Can you work these out from the model? Positions are in its coordinate system, mm. Give positions to 0.01 mm unless a question says otherwise; leave off trailing zeros. Write each loop counter-clockwise with the first axis right and the second up, starting at its lowest first coordinate (ties: lowest second). Pieces come first, ordered by that corner, then holes.
```python
from build123d import *
from OCP.BRepFilletAPI import BRepFilletAPI_MakeChamfer

# Parameters (mm, degrees)
SKETCH1_W           = 990
SKETCH1_H           = 1658
BOSS_EXTRUDE1_DEPTH = 42
SKETCH2_W           = 958
SKETCH2_H           = 1626
CUT_EXTRUDE1_DEPTH  = 2
SKETCH3_W           = 968
SKETCH3_H           = 1636
CUT_EXTRUDE2_DEPTH  = 1932.492687017
SKETCH4_W           = 968
SKETCH4_H           = 1636
SKETCH4_W_2         = 946
SKETCH4_H_2         = 1614
BOSS_EXTRUDE2_DEPTH = 1
CUT_EXTRUDE3_START  = -4
SKETCH5_W           = 980
SKETCH5_H           = 1648
CUT_EXTRUDE3_DEPTH  = 3
CHAMFER1_SIZE       = 3
CHAMFER1_SIZE2      = 5.196152423


with BuildPart() as part:
    # Sketch1 → Boss-Extrude1 (new body)
    with BuildSketch(Plane.XY):
        with Locations((495, 829)):
            Rectangle(SKETCH1_W, SKETCH1_H)
    extrude(amount=BOSS_EXTRUDE1_DEPTH)

    # Sketch2 → Cut-Extrude1 (cut)
    with BuildSketch(Plane.XY.offset(42)):
        with Locations((495, 829)):
            Rectangle(SKETCH2_W, SKETCH2_H)
    extrude(amount=-CUT_EXTRUDE1_DEPTH, mode=Mode.SUBTRACT)

    # Sketch3 → Cut-Extrude2 (cut, through all)
    with BuildSketch(Plane.XY.offset(40)):
        with Locations((495, 829)):
            Rectangle(SKETCH3_W, SKETCH3_H)
    extrude(amount=-CUT_EXTRUDE2_DEPTH, mode=Mode.SUBTRACT)

    # Sketch4 → Boss-Extrude2 (add)
    with BuildSketch(Plane.XY.offset(7)):
        with Locations((495, 829)):
            Rectangle(SKETCH4_W, SKETCH4_H)
        with Locations((495, 829)):
            Rectangle(SKETCH4_W_2, SKETCH4_H_2, mode=Mode.SUBTRACT)
    extrude(amount=BOSS_EXTRUDE2_DEPTH)

    # Sketch5 → Cut-Extrude3 (cut)
    with BuildSketch(Plane(origin=(0, 0, 0), x_dir=(-1, 0, 0), z_dir=(0, 0, -1)).offset(CUT_EXTRUDE3_START)):
        with Locations((-495, 829)):
            Rectangle(SKETCH5_W, SKETCH5_H)
    extrude(amount=-CUT_EXTRUDE3_DEPTH, mode=Mode.SUBTRACT)

    # Chamfer1: one chamfer whose edges measure the first distance from different faces: ONE call of the kernel's chamfer builder (chamfer() names one face for all edges)
    chamfer1_edges_1 = [part.edges().sort_by_distance(p)[0] for p in [
        (495, 1647, 0),
    ]]
    chamfer1_side_1 = [part.faces().sort_by_distance(p)[0] for p in [
        (495, 1647, 2),
    ]]
    chamfer1_edges_2 = [part.edges().sort_by_distance(p)[0] for p in [
        (979, 829, 0),
    ]]
    chamfer1_side_2 = [part.faces().sort_by_distance(p)[0] for p in [
        (979, 829, 2),
    ]]
    chamfer1_edges_3 = [part.edges().sort_by_distance(p)[0] for p in [
        (495, 11, 0),
    ]]
    chamfer1_side_3 = [part.faces().sort_by_distance(p)[0] for p in [
        (495, 11, 2),
    ]]
    chamfer1_edges_4 = [part.edges().sort_by_distance(p)[0] for p in [
        (11, 829, 0),
    ]]
    chamfer1_side_4 = [part.faces().sort_by_distance(p)[0] for p in [
        (11, 829, 2),
    ]]
    chamfer1 = BRepFilletAPI_MakeChamfer(part.part.solid().wrapped)
    for e in chamfer1_edges_1:
        chamfer1.Add(CHAMFER1_SIZE, CHAMFER1_SIZE2, e.wrapped, chamfer1_side_1[0].wrapped)  # the first distance lies on this face
    for e in chamfer1_edges_2:
        chamfer1.Add(CHAMFER1_SIZE, CHAMFER1_SIZE2, e.wrapped, chamfer1_side_2[0].wrapped)  # the first distance lies on this face
    for e in chamfer1_edges_3:
        chamfer1.Add(CHAMFER1_SIZE, CHAMFER1_SIZE2, e.wrapped, chamfer1_side_3[0].wrapped)  # the first distance lies on this face
    for e in chamfer1_edges_4:
        chamfer1.Add(CHAMFER1_SIZE, CHAMFER1_SIZE2, e.wrapped, chamfer1_side_4[0].wrapped)  # the first distance lies on this face
    add(Compound.cast(chamfer1.Shape()), mode=Mode.REPLACE)


solid = part.part
```
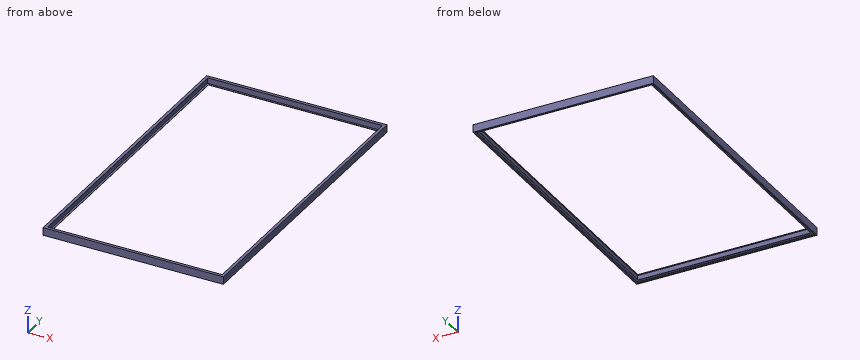
1) Suppose I cut it at B-B on y = 1087. Write out the boundary of the cut face in (x, z), plus the area to 3 significant figures.
Values follow:
outline: (0, 0) - (5.8, 0) - (11, 3) - (11, 4) - (5, 4) - (5, 7) - (22, 7) - (22, 8) - (11, 8) - (11, 40) - (16, 40) - (16, 42) - (0, 42) - close; (968, 7) - (985, 7) - (985, 4) - (979, 4) - (979, 3) - (984.2, 0) - (990, 0) - (990, 42) - (974, 42) - (974, 40) - (979, 40) - (979, 8) - (968, 8) - close
area: 914 mm2
2) Please list where these lines run through material, in increasing order: L1, parallel to X at y = 1104.5, z = 5.5; L2, parallel to X at y = 72.5, z = 22; L3, parallel to Y at x = 57, z = 10.
Values follow:
L1: x = 0 to 5, 985 to 990
L2: x = 0 to 11, 979 to 990
L3: y = 0 to 11, 1647 to 1658
3) Suppose I cut it at A-A on z = 30. Write out the boundary of the cut face in (x, y), plus the area to 3 significant figures.
Values follow:
outline: (0, 0) - (990, 0) - (990, 1658) - (0, 1658) - close; hole (11, 11) - (979, 11) - (979, 1647) - (11, 1647) - close
area: 57,800 mm2
4) Suppose I cut it at C-C on x = 857. Write out the boundary of the cut face in (y, z), plus the area to 3 significant figures.
Values follow:
outline: (0, 0) - (5.8, 0) - (11, 3) - (11, 4) - (5, 4) - (5, 7) - (22, 7) - (22, 8) - (11, 8) - (11, 40) - (16, 40) - (16, 42) - (0, 42) - close; (1636, 7) - (1653, 7) - (1653, 4) - (1647, 4) - (1647, 3) - (1652.2, 0) - (1658, 0) - (1658, 42) - (1642, 42) - (1642, 40) - (1647, 40) - (1647, 8) - (1636, 8) - close
area: 914 mm2
